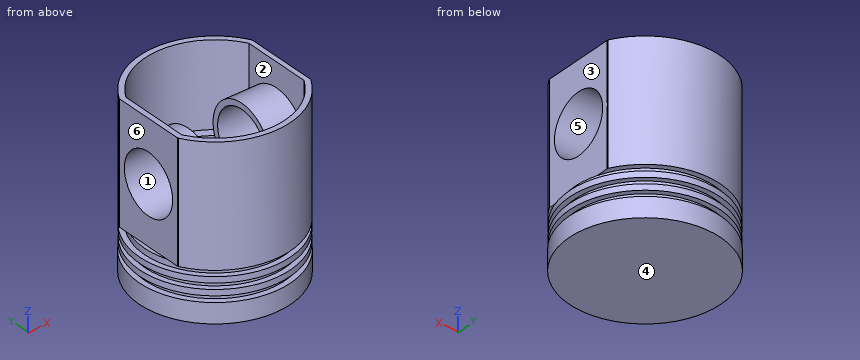
```python
from build123d import *

# Parameters (mm, degrees)
F0_R      = 48.4220762832
F1_DEPTH  = 76.2
F2_R      = 44.958
F3_DEPTH  = 71.12
F4_R      = 44.958
F5_DEPTH  = 3.81
F6_R      = 48.26
F7_DEPTH  = 3.81
F8_R      = 44.958
F9_DEPTH  = 3.81
F10_R     = 48.26
F11_DEPTH = 3.81
F12_R     = 44.958
F13_DEPTH = 3.81
F14_R     = 48.4881238819
F15_DEPTH = 12.7
F16_R     = 44.958
F16_R_2   = 39.5280108498
F17_DEPTH = 17.78
F18_W     = 24.8659998178
F18_H     = 81.0338929296
F19_DEPTH = 76.201
F20_W     = 28.6690369248
F20_H     = 83.0816850066
F21_DEPTH = 76.201
F22_W     = 3.4077020206
F22_H     = 45.72
F23_DEPTH = 76.2
F24_W     = 3.1630169219
F24_H     = 45.72
F25_DEPTH = 76.2
F26_R     = 22.7868641695
F27_DEPTH = 25.4
F28_R     = 19.05
F29_DEPTH = 25.4
F31_DEPTH = 25.4
F32_R     = 19.05
F33_DEPTH = 25.4


with BuildPart() as f1:
    # F0 (on Top) → F1 (new body)
    with BuildSketch(Plane.XY):
        Circle(F0_R)
    extrude(amount=F1_DEPTH)

    # F2 (on face) → F3 (cut)
    with BuildSketch(Plane.XY.offset(76.2)):
        Circle(F2_R)
    extrude(amount=-F3_DEPTH, mode=Mode.SUBTRACT)

    # F4 (on Top) → F5 (join)
    with BuildSketch(Plane.XY):
        Circle(F4_R)
    extrude(amount=-F5_DEPTH)

    # F6 (on face) → F7 (join)
    with BuildSketch(Plane(origin=(0, 0, -3.81), x_dir=(1, 0, 0), z_dir=(0, 0, -1))):
        Circle(F6_R)
    extrude(amount=F7_DEPTH)

    # F8 (on face) → F9 (join)
    with BuildSketch(Plane(origin=(0, 0, -7.62), x_dir=(1, 0, 0), z_dir=(0, 0, -1))):
        Circle(F8_R)
    extrude(amount=F9_DEPTH)

    # F10 (on face) → F11 (join)
    with BuildSketch(Plane(origin=(0, 0, -11.43), x_dir=(1, 0, 0), z_dir=(0, 0, -1))):
        Circle(F10_R)
    extrude(amount=F11_DEPTH)

    # F12 (on face) → F13 (join)
    with BuildSketch(Plane(origin=(0, 0, -15.24), x_dir=(1, 0, 0), z_dir=(0, 0, -1))):
        Circle(F12_R)
    extrude(amount=F13_DEPTH)

    # F14 (on face) → F15 (join)
    with BuildSketch(Plane(origin=(0, 0, -19.05), x_dir=(1, 0, 0), z_dir=(0, 0, -1))):
        Circle(F14_R)
    extrude(amount=F15_DEPTH)

    # F16 (on face) → F17 (join)
    with BuildSketch(Plane.XY.offset(5.08)):
        Circle(F16_R)
        Circle(F16_R_2, mode=Mode.SUBTRACT)
    extrude(amount=F17_DEPTH)

    # F18 (on Top) → F19 (cut, through all)
    with BuildSketch(Plane.XY):
        with Locations((-54.7783300281, -4.0224418044)):
            Rectangle(F18_W, F18_H)
    extrude(amount=F19_DEPTH, mode=Mode.SUBTRACT)

    # F20 (on Top) → F21 (cut, through all)
    with BuildSketch(Plane.XY):
        with Locations((56.8261183798, -3.8761682808)):
            Rectangle(F20_W, F20_H)
    extrude(amount=F21_DEPTH, mode=Mode.SUBTRACT)

    # F22 (on Top) → F23 (join)
    with BuildSketch(Plane.XY):
        with Locations((-40.8826228231, 0.0731358305)):
            Rectangle(F22_W, F22_H)
    extrude(amount=F23_DEPTH)

    # F24 (on Top) → F25 (join)
    with BuildSketch(Plane.XY):
        with Locations((40.9449934959, -0.2194056287)):
            Rectangle(F24_W, F24_H)
    extrude(amount=F25_DEPTH)

    # F26 (on face) → F27 (join)
    with BuildSketch(Plane(origin=(-42.5864738334, 0, 0), x_dir=(0, -1, 0), z_dir=(-1, 0, 0))):
        with Locations((0, 37.2258611023)):
            Circle(F26_R)
    extrude(amount=-F27_DEPTH)

    # F28 (on face) → F29 (cut)
    with BuildSketch(Plane.YZ.offset(-17.1864738334)):
        with Locations((0, 37.2258611023)):
            Circle(F28_R)
    extrude(amount=-F29_DEPTH, mode=Mode.SUBTRACT)

    # F30 (on face) → F31 (join)
    with BuildSketch(Plane.YZ.offset(42.5265019569)):
        with BuildLine():
            Line((22.6405943713, 36.7378248993), (22.6405943713, 39.4621751007))
            ThreePointArc((22.6405943713, 39.4621751007), (-22.6815350999, 38.1), (22.6405943713, 36.7378248993))
        make_face()
        with BuildLine():
            ThreePointArc((22.6405943713, 36.7378248993), (22.6712976074, 37.4186048965), (22.6815350999, 38.1))
            ThreePointArc((22.6815350999, 38.1), (22.6712976074, 38.7813951035), (22.6405943713, 39.4621751007))
            Line((22.6405943713, 39.4621751007), (22.6405943713, 36.7378248993))
        make_face()
    extrude(amount=-F31_DEPTH)

    # F32 (on face) → F33 (cut)
    with BuildSketch(Plane(origin=(17.1265019569, 0, 0), x_dir=(0, -1, 0), z_dir=(-1, 0, 0))):
        with Locations((0, 38.1)):
            Circle(F32_R)
    extrude(amount=-F33_DEPTH, mode=Mode.SUBTRACT)


solid = f1.part
```
Geometry: final body of the model. Coordinates: model frame, mm. Face numbers are marked on the shaded views. A direction names the side the tool comes from. Round coordinates to 2 decimals unless told otherwise and drop trailing zeros. Use one line per item in the form item = value. Start each with the question number.
1) Line query: L1, parallel to Z at x = -35.25, y = 0; L2, parallel to Z at x = 26.5, y = 0; L3, parallel to X at y = -20, z = 61. Output: solid intervals per line, ascending.
2) First-contact query: P1, Ø8.5, axis at x = 12.5, y = 31.5, coming from the +Z side; P2, Ø2, axis at y = 18, z = 59, coming from the +X side; P3, Ø12, axis at x = -5.5, z = 1, coming from the -Y side; P4, Ø13.5, axis at y = -1, z = 44, coming from the -X side. Flat tips, straight axial feed; report the tip coordinate or a pass-through.
3) Access query for the marked faces 1, 2 and 3. Directions: +Z, -Z, +X, -X, +Y, -Y. A direction counts if a zero-diameter tool reaches every point of the face in a straight line with its end or side. Return the directions, or none.
4) Section B-B on y = 0. Give the number of separate pieces and of enclosed holes in the cut face, then the cut area to 3 significant figures.
5) Draft query along Z for the marked faces 4, 5 and 6. Return one class per face: released by +Z, released by -Z, zero draft, split by the parting line, or undercut.
Response:
q1.L1 = -31.75 to 5.08, 14.44 to 18.18, 56.28 to 60.01
q1.L2 = -31.75 to 5.08, 15.42 to 19.05, 57.15 to 60.78
q1.L3 = -42.59 to -39.18, 39.36 to 42.53
q2.P1 = 5.08
q2.P2 = 42.53
q2.P3 = -48.42
q2.P4 = through
q3.face_1 = -X
q3.face_2 = +Z
q3.face_3 = +Z, +X, +Y, -Y
q4.separate_pieces = 3
q4.enclosed_holes = 0
q4.area = 3,970 mm^2
q5.face_4 = released by -Z
q5.face_5 = undercut
q5.face_6 = zero draft
